Work out the finished part from the listing and answer in its coordinate system (mm). Face numbers are marked on the shaded views. A direction names the side the tool comes from. Give positions to 0.01 mm unless a question says otherwise; leave off trailing zeros. Order: outer loops, then holes, each group sorted by start corner. A loop starts at its lowest first (then second) coordinate and runs counter-clockwise, first axis right, second up. Notation, with made-up numbers: (40.25, -21.5) - (68.25, -21.5) arc R29 cw to (68.25, 7.5) - close; hole circle Ø11 at (-19, 59.25). An arc over 180 degrees is marked (long way). Return JSON: item names as keys, results as strings. Group by question number.
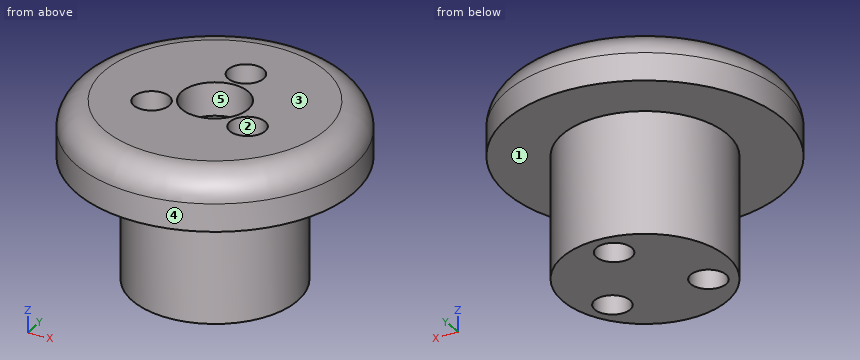
from build123d import *

# Parameters (mm, degrees)
SKETCH2_R           = 7.45
BOSS_EXTRUDE1_DEPTH = 11
SKETCH3_R           = 12.5
BOSS_EXTRUDE2_DEPTH = 5
SKETCH4_R           = 1.6
CUT_EXTRUDE1_DEPTH  = 24.843238035
FILLET2_R           = 2.5
SKETCH5_R           = 3
CUT_EXTRUDE2_DEPTH  = 3


with BuildPart() as part:
    # Sketch2 → Boss-Extrude1 (new body)
    with BuildSketch(Plane.XY):
        Circle(SKETCH2_R)
    extrude(amount=BOSS_EXTRUDE1_DEPTH)

    # Sketch3 → Boss-Extrude2 (add)
    with BuildSketch(Plane.XY.offset(11)):
        Circle(SKETCH3_R)
    extrude(amount=BOSS_EXTRUDE2_DEPTH)

    # Sketch4 → Cut-Extrude1 (cut, through all)
    with BuildSketch(Plane.XY.offset(16)):
        with Locations((0, 5)):
            Circle(SKETCH4_R)
        with Locations((4.330127019, -2.5)):
            Circle(SKETCH4_R)
        with Locations((-4.330127019, -2.5)):
            Circle(SKETCH4_R)
    extrude(amount=-CUT_EXTRUDE1_DEPTH, mode=Mode.SUBTRACT)

    # Fillet2
    fillet2_edges = [part.edges().sort_by_distance(p)[0] for p in [
        (-12.5, 0, 16),
    ]]
    fillet(fillet2_edges, radius=FILLET2_R)

    # Sketch5 → Cut-Extrude2 (cut)
    with BuildSketch(Plane.XY.offset(16)):
        Circle(SKETCH5_R)
    extrude(amount=-CUT_EXTRUDE2_DEPTH, mode=Mode.SUBTRACT)


solid = part.part
1. Determine the mould class of the marked faces 3, 4 and 5 for opening direction Y: released by +Y, released by -Y, zero draft, split by the parting line, or undercut.
2. The part is cut by section C-C (y = 0). Give the vertices of the cut face in (x, z).
3. Each of these flat-tipped pins is pushed along its axis until it touches: pin 1 (3 mm diameter, centred on x = 0.5, y = 0, fed in from +Z); pin 2 (4 mm diameter, centred on x = -4.33, y = -2.5, fed in from +Z); pin 3 (3 mm diameter, centred on y = 3, z = 14, fed in from +X); pin 4 (5 mm diameter, centred on x = -3.5, z = 5.5, fed in from +Y). Where does it stop, or does it pass through?
4. The part is cut by section B-B (z = 10). Give the vertices of the cut face in (x, y), and give its area (3 significant figures).
5. The part is cut by section A-A (x = 0). Give the vertices of the cut face in (y, z).
6. The part is cut by section D-D (y = -2.5). State how many separate pieces and enclosed holes the cut face has, and give its area (3 significant figures).
7. Consider probe 1 along Y at (x, z) = (0, 4.25); probe 2 along Y at (x, z) = (-4.5, 5); probe 3 along Z at (x, y) = (9, -1). Determine where each line is inside the solid, lowest interval first. Write a range as from..to.
8. A tool of negligible diameter and unlimited length cuts with its end or side. For the marked faces 1 and 2, from which of +Z, -Z, +X, -X, +Y, -Y can it reach the whole face along a straight path? Write none if from no direction.
Answers:
{
 "1": {"face 3": "zero draft", "face 4": "split by the parting line", "face 5": "undercut"},
 "2": {"outline": "(-12.5, 11) - (-7.45, 11) - (-7.45, 0) - (7.45, 0) - (7.45, 11) - (12.5, 11) - (12.5, 13.5) arc R2.5 ccw to (10, 16) - (3, 16) - (3, 13) - (-3, 13) - (-3, 16) - (-10, 16) arc R2.5 ccw to (-12.5, 13.5) - close"},
 "3": {"pin 1": "stops at z = 13", "pin 2": "stops at z = 16", "pin 3": "stops at x = 12.4", "pin 4": "stops at y = 7.38"},
 "4": {"outline": "circle Ø14.9 at (0, 0); hole circle Ø3.2 at (-4.33, -2.5); hole circle Ø3.2 at (0, 5); hole circle Ø3.2 at (4.33, -2.5)", "area": "150 mm^2"},
 "5": {"outline": "(-12.5, 11) - (-7.45, 11) - (-7.45, 0) - (3.4, 0) - (3.4, 16) - (3, 16) - (3, 13) - (-3, 13) - (-3, 16) - (-10, 16) arc R2.5 ccw to (-12.5, 13.5) - close; (6.6, 0) - (7.45, 0) - (7.45, 11) - (12.5, 11) - (12.5, 13.5) arc R2.5 ccw to (10, 16) - (6.6, 16) - close"},
 "6": {"separate pieces": "3", "enclosed holes": "0", "area": "162 mm^2"},
 "7": {"probe 1": "y = -7.45..3.4, 6.6..7.45", "probe 2": "y = -5.94..-4.09, -0.91..5.94", "probe 3": "z = 11..16"},
 "8": {"face 1": "-Z", "face 2": "+Z, -Z"}
}
